CAD build for the part. Positions are in the model's coordinates, mm. A direction names the side the tool comes from. Give positions to 0.01 mm unless a question says otherwise; leave off trailing zeros. Order: outer loops, then holes, each group sorted by start corner. A loop starts at its lowest first (then second) coordinate and runs counter-clockwise, first axis right, second up.
```python
from build123d import *

# Parameters (mm, degrees)
SKETCH1_R                      = 14
BOSS_EXTRUDE1_DEPTH            = 1.75
M2_5_CLEARANCE_HOLE1_D         = 3.1
M2_5_CLEARANCE_HOLE1_DEPTH     = 6
M2_5_CLEARANCE_HOLE1_TIP       = 0.931333959
SKETCH9_R                      = 8
BOSS_EXTRUDE2_DEPTH            = 10
SKETCH7_R                      = 5
CUT_EXTRUDE1_DEPTH             = 24.963513933
M5_CLEARANCE_HOLE1_D           = 5.3
M5_CLEARANCE_HOLE1_DEPTH       = 25.4
M5_CLEARANCE_HOLE1_CSINK_D     = 5.35
M5_CLEARANCE_HOLE1_CSINK_ANGLE = 90
M5_CLEARANCE_HOLE1_TIP         = 1.59228064


with BuildPart() as part:
    # Sketch1 → Boss-Extrude1 (new, symmetric)
    with BuildSketch(Plane(origin=(0, 0, 0), x_dir=(1, 0, 0), z_dir=(0, 1, 0))):
        with Locations(Location((0, 0, 0), (0, 0, 270))):
            Circle(SKETCH1_R)
    extrude(amount=BOSS_EXTRUDE1_DEPTH, both=True)

    # M2.5 Clearance Hole1
    with Locations(Plane(origin=(0, 1.75, 0), x_dir=(1, 0, 0), z_dir=(0, 1, 0))):
        with Locations((-11, 0), (-7.778174593, 7.778174593), (0, 11), (7.778174593, 7.778174593), (11, 0), (7.778174593, -7.778174593), (0, -11), (-7.778174593, -7.778174593)):
            Hole(M2_5_CLEARANCE_HOLE1_D / 2, depth=M2_5_CLEARANCE_HOLE1_DEPTH)
            with Locations((0, 0, -(M2_5_CLEARANCE_HOLE1_DEPTH + M2_5_CLEARANCE_HOLE1_TIP / 2))):  # 118° drill point
                Cone(0, M2_5_CLEARANCE_HOLE1_D / 2, M2_5_CLEARANCE_HOLE1_TIP, mode=Mode.SUBTRACT)

    # Sketch9 → Boss-Extrude2 (add)
    with BuildSketch(Plane(origin=(0, 1.75, 0), x_dir=(1, 0, 0), z_dir=(0, 1, 0))):
        with Locations(Location((0, 0, 0), (0, 0, 270))):
            Circle(SKETCH9_R)
    extrude(amount=BOSS_EXTRUDE2_DEPTH)

    # Sketch7 → Cut-Extrude1 (cut, through all)
    with BuildSketch(Plane.XZ.offset(1.75)):
        with Locations(Location((0, 0, 0), (0, 0, 270))):
            Circle(SKETCH7_R)
    extrude(amount=-CUT_EXTRUDE1_DEPTH, mode=Mode.SUBTRACT)

    # M5 Clearance Hole1
    with Locations(Plane(origin=(8, 0, 0), x_dir=(0, 0, -1), z_dir=(1, 0, 0))):
        with Locations((0, 6.75)):
            CounterSinkHole(M5_CLEARANCE_HOLE1_D / 2, M5_CLEARANCE_HOLE1_CSINK_D / 2, depth=M5_CLEARANCE_HOLE1_DEPTH, counter_sink_angle=M5_CLEARANCE_HOLE1_CSINK_ANGLE)
            with Locations((0, 0, -(M5_CLEARANCE_HOLE1_DEPTH + M5_CLEARANCE_HOLE1_TIP / 2))):  # 118° drill point
                Cone(0, M5_CLEARANCE_HOLE1_D / 2, M5_CLEARANCE_HOLE1_TIP, mode=Mode.SUBTRACT)


solid = part.part
```
Item 1: Slice it at A-A (x = 0). Give the cut face in (y, z).
Item 2: Slice it at D-D (x = 10.75). Give the cut face in (y, z), and give its area (3 significant figures).
Item 3: Slice it at C-C (y = 4.75). Give the cut face in (x, z).
Item 4: Wall check: L1, parallel to Y at x = -5.4, z = 0; L2, parallel to Z at x = 0.25, y = 0; L3, parallel to X at y = 11.25, z = 0. Give the ranges that are in metal, low to high.
Item 5: Slice it at B-B (z = 0). State how many separate pieces and enclosed holes the cut face has, and give its area (3 significant figures).
Item 6: Tool access for faces 4 (the face through (-7.1, 6.68, 3.69)), 5 (the face through (-9.77, -0.02, 0.94)): list every direction of +Z, -Z, +X, -X, +Y, -Y with a clear straight run to the whole face (end or side of a thin tool).
Item 7: Drop flat-ended pins along their axis: pin 1 Ø3.5 at (x, z) = (0, -11) entering from +Y; pin 2 Ø2.5 at (x, z) = (-7.78, 7.78) entering from +Y; pin 3 Ø8 at (x, y) = (-5.5, 0) entering from -Z; pin 4 Ø1 at (y, z) = (0.5, -3) entering from +X (3 decimals). Give the stop position or say it passes through.
Item 8: Two-plate mould, pull along Y, no slides. Class faces 1 (the face through (-6, 1.75, 6)), 2 (the face through (6.1, 9, 1.4)), 3 (the face through (-13.67, 0.02, -3.03)): released by +Y, released by -Y, zero draft, split by the parting line, or undercut.
A:
1. outline: (-1.75, -14) - (1.75, -14) - (1.75, -12.55) - (-1.75, -12.55) - close; (-1.75, -9.45) - (1.75, -9.45) - (1.75, -8) - (11.75, -8) - (11.75, -5) - (-1.75, -5) - close; (-1.75, 5) - (11.75, 5) - (11.75, 8) - (1.75, 8) - (1.75, 9.45) - (-1.75, 9.45) - close; (-1.75, 12.55) - (1.75, 12.55) - (1.75, 14) - (-1.75, 14) - close
2. outline: (-1.75, -8.97) - (1.75, -8.97) - (1.75, -1.53) - (-1.75, -1.53) - close; (-1.75, 1.53) - (1.75, 1.53) - (1.75, 8.97) - (-1.75, 8.97) - close
2. area: 52.1 mm2
3. outline: (-7.81, -1.74) arc R8 ccw to (7.81, -1.74) - (4.69, -1.74) arc R5 cw to (-4.69, -1.74) - close; (-7.81, 1.74) - (-4.69, 1.74) arc R5 cw to (4.69, 1.74) - (7.81, 1.74) arc R8 ccw to start
4. L1: y = -1.75 to 4.1, 9.4 to 11.75
4. L2: z = -14 to -12.53, -9.47 to -4.99, 4.99 to 9.47, 12.53 to 14
4. L3: x = -8 to -5, 5 to 8
5. separate pieces: 6
5. enclosed holes: 0
5. area: 69.5 mm2
6. face 4: +Y
6. face 5: +Y, -Y
7. pin 1: stops at y = 1.75
7. pin 2: passes through
7. pin 3: stops at z = -13.92
7. pin 4: stops at x = 13.775
8. face 1: released by +Y
8. face 2: undercut
8. face 3: zero draft
